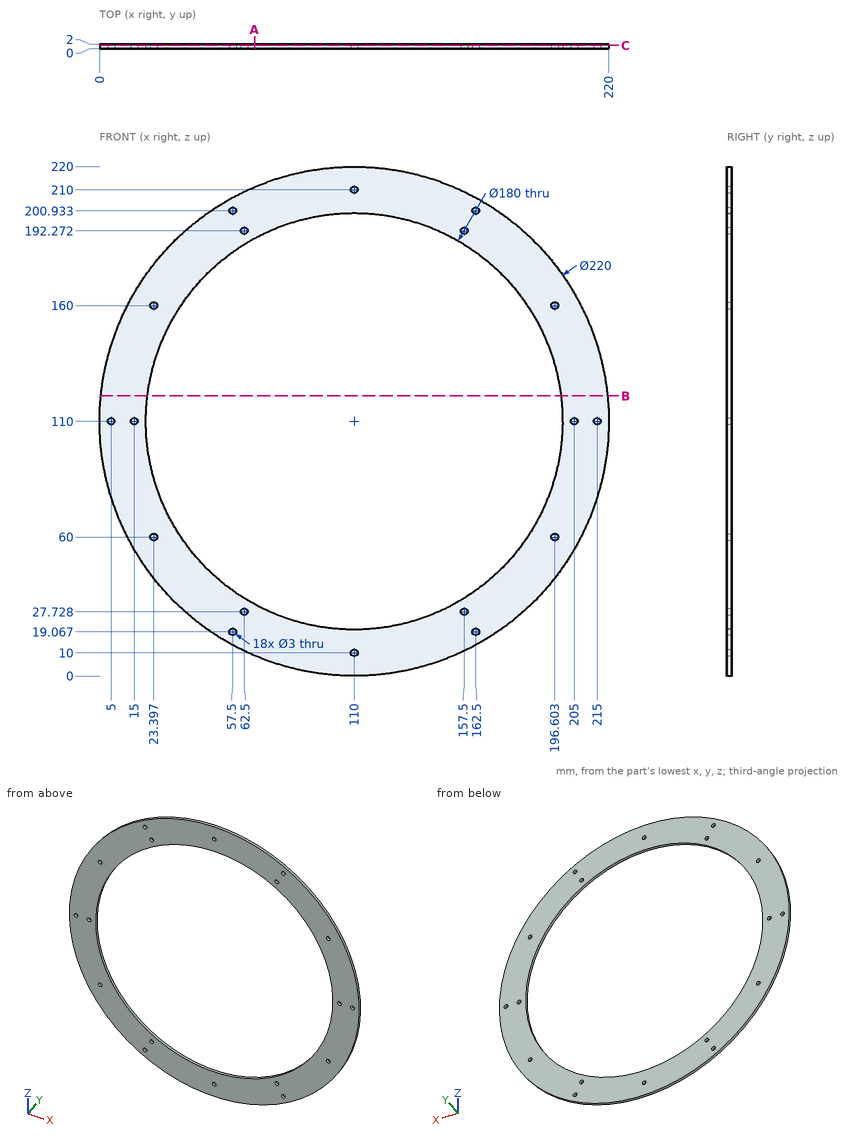
Geometry check sheet. Reference: drawing and pictorial views, mm from the part's lowest x, y, z. Give positions to 0.01 mm unless a question says otherwise; leave off trailing zeros. Order: outer loops, then holes, each group sorted by start corner. A loop starts at its lowest first (then second) coordinate and runs counter-clockwise, first axis right, second up. Notation, with made-up numbers: M 39,-26 L 83,-26 A33 ccw 83,2 Z; hole C 14.5,63.25 d4. An arc over 180 degrees is marked long. Answer in a Markdown table with one row per item.
1) Thickness scan on L1, parallel to X at y = 1.6, z = 160.5 (1 decimal); L2, parallel to Z at x = 163, y = 0.45 (1 decimal); L3, parallel to Z at x = 98, y = 1.25. Record the ranges inside material, lowest first. Write a range as [from, to].
Filled sheet:
| item | result |
|---|---|
| L1 | x = [12.3, 22], [24.8, 35.5], [184.5, 195.2], [198, 207.7] |
| L2 | z = [13.6, 17.7], [20.5, 37.3], [182.7, 199.5], [202.3, 206.4] |
| L3 | z = [0.66, 20.8], [199.2, 219.34] |
2) Cross-section at C-C, the plane y = 1.45. Count the separate pieces of the cut face and the enclosed holes in it, plus the area to 3 significant figures.
Filled sheet:
| item | result |
|---|---|
| separate pieces | 1 |
| enclosed holes | 19 |
| area | 12,400 mm2 |
3) Cross-section at B-B, the plane z = 121. Enter the section's corners in (x, y) (1 decimal).
Filled sheet:
| item | result |
|---|---|
| outline | M 0.6,0 L 20.7,0 L 20.7,2 L 0.6,2 Z; M 199.3,0 L 219.4,0 L 219.4,2 L 199.3,2 Z |
4) Cross-section at A-A, the plane x = 67. Enter the section's corners in (y, z).
Filled sheet:
| item | result |
|---|---|
| outline | M 0,8.75 L 2,8.75 L 2,30.94 L 0,30.94 Z; M 0,189.06 L 2,189.06 L 2,211.25 L 0,211.25 Z |
5) Gauge pin test, flat end, axial feed: P1, Ø1.8, axis at x = 157.5, z = 27.73, coming from the +Y side. Record the tip position at first contact, or that the pin passes through.
Filled sheet:
| item | result |
|---|---|
| P1 | passes through |
